Geometry: final body of the model. Coordinates: model frame, mm. A direction names the side the tool comes from. Give positions to 0.01 mm unless a question says otherwise; leave off trailing zeros. Order: outer loops, then holes, each group sorted by start corner. A loop starts at its lowest first (then second) coordinate and runs counter-clockwise, first axis right, second up. Notation, with made-up numbers: (83.25, -25.5) - (110.25, -25.5) arc R16 cw to (110.25, -8.5) - close; hole circle Ø5 at (52, 7.25). An arc over 180 degrees is marked (long way). Use one line per item in the form item = value.
from build123d import *

# Parameters (mm, degrees)
F0_R      = 50
F1_DEPTH  = 80
F2_R      = 25
F3_DEPTH  = 50
F4_R      = 20
F5_DEPTH  = 40
F6_R      = 25
F7_DEPTH  = 20
F8_R      = 20
F9_DEPTH  = 20
F10_R     = 15
F11_DEPTH = 20
F12_R     = 10
F13_DEPTH = 20
F14_R     = 2.5
F15_DEPTH = 20


with BuildPart() as f1:
    # F0 (on Front) → F1 (new body)
    with BuildSketch(Plane.XZ):
        Circle(F0_R)
    extrude(amount=F1_DEPTH)

    # F2 (on face) → F3 (join)
    with BuildSketch(Plane.XZ.offset(80)):
        Circle(F2_R)
    extrude(amount=F3_DEPTH)

    # F4 (on face) → F5 (cut)
    with BuildSketch(Plane.XZ.offset(130)):
        Circle(F4_R)
    extrude(amount=-F5_DEPTH, mode=Mode.SUBTRACT)

    # F6 (on face) → F7 (join)
    with BuildSketch(Plane(origin=(0, 0, 0), x_dir=(-1, 0, 0), z_dir=(0, 1, 0))):
        Circle(F6_R)
    extrude(amount=F7_DEPTH)

    # F8 (on face) → F9 (join)
    with BuildSketch(Plane(origin=(0, 20, 0), x_dir=(-1, 0, 0), z_dir=(0, 1, 0))):
        Circle(F8_R)
    extrude(amount=F9_DEPTH)

    # F10 (on face) → F11 (join)
    with BuildSketch(Plane(origin=(0, 40, 0), x_dir=(-1, 0, 0), z_dir=(0, 1, 0))):
        Circle(F10_R)
    extrude(amount=F11_DEPTH)

    # F12 (on face) → F13 (join)
    with BuildSketch(Plane(origin=(0, 60, 0), x_dir=(-1, 0, 0), z_dir=(0, 1, 0))):
        Circle(F12_R)
    extrude(amount=F13_DEPTH)

    # F14 (on face) → F15 (join)
    with BuildSketch(Plane(origin=(0, 80, 0), x_dir=(-1, 0, 0), z_dir=(0, 1, 0))):
        Circle(F14_R)
    extrude(amount=F15_DEPTH)


solid = f1.part
(1) Contact query for flat-ended pins moving along their axis: pin 1 Ø1.5 at (x, y) = (34.5, -34) entering from -Z; pin 2 Ø4 at (x, y) = (0, -105) entering from -Z; pin 3 Ø3 at (x, y) = (4.5, 65) entering from +Z. Output: stop coordinate, or through.
Computed values:
pin_1 = -36.89
pin_2 = -25
pin_3 = 9.54
(2) Reachability of faces 4 (the face through (23.846, -104.65, 7.509)), 5 (the face through (-2, 80, -2)), 6 (the face through (47.69, -39.44, 15.02)) from +Z, -Z, +X, -X, +Y, -Y: full face, straight path, thin tool, end or side. Return the list, or none.
Computed values:
face_4 = -Y
face_5 = +Y
face_6 = +Y, -Y
(3) Pull-direction query (X, two-part tool) for faces 1 (the face through (-22.9, -80, -10.4)), 2 (the face through (-4.336, -110.28, -19.524)), 3 (the face through (0.54, 89.86, -2.44)); classes: released by +X, released by -X, zero draft, split by the parting line, or undercut.
Computed values:
face_1 = zero draft
face_2 = undercut
face_3 = split by the parting line
(4) Ray query, line 1 along Z through (x, y) = (0, -113); line 2 along Y through (x, z) = (10, 34.5); line 3 along Y through (x, z) = (-3, -3.5). Return the intervals inside material, ascending.
Computed values:
line_1 = -25 to -20, 20 to 25
line_2 = -80 to 0
line_3 = -90 to 80
(5) Cut plane C-C on y = -13. Output: boundary loops of the cut face in (x, z), plus the area to 3 significant figures.
Computed values:
outline = circle Ø100 at (0, 0)
area = 7,850 mm²
(6) Cut plane D-D on z = 36.5. Output: boundary loops of the cut face in (x, y), plus the area to 3 significant figures.
Computed values:
outline = (-34.17, -80) - (34.17, -80) - (34.17, 0) - (-34.17, 0) - close
area = 5,470 mm²
